Can you work these out from the model? Positions are in its coordinate system, mm. A direction names the side the tool comes from. Give positions to 0.01 mm unless a question says otherwise; leave off trailing zeros. Order: outer loops, then holes, each group sorted by start corner. A loop starts at its lowest first (then second) coordinate and runs counter-clockwise, first axis right, second up. Notation, with made-up numbers: (10.25, -27) - (22.25, -27) arc R17 cw to (22.25, -22) - close; hole circle Ø10 at (-7.75, -37.5). An arc over 180 degrees is marked (long way). Return JSON: item names as keys, results as strings.
```python
from build123d import *

# Parameters (mm, degrees)
SKETCH1_R           = 15
BOSS_EXTRUDE1_DEPTH = 6
SKETCH5_R           = 5.35
CUT_EXTRUDE2_DEPTH  = 11.5
CUT_EXTRUDE3_START  = -1
CUT_EXTRUDE3_DEPTH  = 3
SKETCH7_R           = 3.2
CUT_EXTRUDE4_DEPTH  = 2.5


with BuildPart() as part:
    # Sketch1 → Boss-Extrude1 (new body)
    with BuildSketch(Plane(origin=(0, 0, 0), x_dir=(0, 1, 0), z_dir=(0, 0, 1))):
        with Locations(Location((0, 0, 0), (0, 0, 270))):
            Circle(SKETCH1_R)
    extrude(amount=BOSS_EXTRUDE1_DEPTH)

    # Sketch5 → Cut-Extrude2 (cut)
    with BuildSketch(Plane(origin=(0, 0, 0), x_dir=(1, 0, 0), z_dir=(0, 0, -1))):
        with Locations(Location((0, 0, 0), (0, 0, 180))):
            Circle(SKETCH5_R)
    extrude(amount=-CUT_EXTRUDE2_DEPTH, mode=Mode.SUBTRACT)

    # Sketch2 → Cut-Extrude3 (cut)
    with BuildSketch(Plane.XY.offset(6).offset(CUT_EXTRUDE3_START)):
        Polygon((8.873853267, -8.742858672), (12.008464346, -6.786446977), (11.881467657, -3.093588305), (8.619859889, -1.357141328), (5.485248811, -3.313553023), (5.6122455, -7.006411695), align=None)
        Polygon((3.134611078, 12.056411695), (-0.126996689, 13.792858672), (-3.261607767, 11.836446977), (-3.134611078, 8.143588305), (0.126996689, 6.407141328), (3.261607767, 8.363553023), align=None)
        Polygon((-12.008464346, -3.313553023), (-11.881467657, -7.006411695), (-8.619859889, -8.742858672), (-5.485248811, -6.786446977), (-5.6122455, -3.093588305), (-8.873853267, -1.357141328), align=None)
    extrude(amount=-CUT_EXTRUDE3_DEPTH, mode=Mode.SUBTRACT)

    # Sketch7 → Cut-Extrude4 (cut)
    with BuildSketch(Plane.XY.offset(6)):
        with Locations((8.746856578, -5.05)):
            Circle(SKETCH7_R)
        with Locations((0, 10.1)):
            Circle(SKETCH7_R)
        with Locations((-8.746856578, -5.05)):
            Circle(SKETCH7_R)
    extrude(amount=-CUT_EXTRUDE4_DEPTH, mode=Mode.SUBTRACT)


solid = part.part
```
1. For pin 1 Ø3 at (x, z) = (-4.5, 4.5) entering from +Y; pin 2 Ø3 at (x, z) = (-8.5, 1) entering from -Y; pin 3 Ø2 at (y, z) = (-11.5, 3) entering from -X, each with a flat end and sliding along its axis, tell me the tip position at first contact or that it passes through.
Checks:
{"pin 1": "y = 14.7", "pin 2": "y = -13.27", "pin 3": "x = -10.71"}
2. Suppose I cut it at B-B (z = 5.55). List the corners of the cut face in (x, y) for me, plus the area to 3 significant figures.
Checks:
{"outline": "circle Ø30 at (0, 0); hole circle Ø6.4 at (-8.75, -5.05); hole circle Ø10.7 at (0, 0); hole circle Ø6.4 at (0, 10.1); hole circle Ø6.4 at (8.75, -5.05)", "area": "520 mm^2"}
3. Suppose I cut it at D-D (x = -6). List the corners of the cut face in (y, z) for me, plus the area to 3 significant figures.
Checks:
{"outline": "(-13.75, 0) - (13.75, 0) - (13.75, 6) - (-3.41, 6) - (-3.41, 5) - (-2.89, 5) - (-2.89, 2) - (-7.11, 2) - (-7.11, 5) - (-6.69, 5) - (-6.69, 6) - (-13.75, 6) - close", "area": "149 mm^2"}
4. Suppose I cut it at C-C (x = 1). List the corners of the cut face in (y, z) for me.
Checks:
{"outline": "(-14.97, 0) - (-5.26, 0) - (-5.26, 6) - (-14.97, 6) - close; (5.26, 0) - (14.97, 0) - (14.97, 6) - (13.14, 6) - (13.14, 5) - (13.19, 5) - (13.19, 2) - (6.95, 2) - (6.95, 5) - (7.06, 5) - (7.06, 6) - (5.26, 6) - close"}
5. Suppose I cut it at A-A (y = 0). List the corners of the cut face in (x, z) for me.
Checks:
{"outline": "(-15, 0) - (-5.35, 0) - (-5.35, 6) - (-15, 6) - close; (5.35, 0) - (15, 0) - (15, 6) - (5.35, 6) - close"}
6. If I drill on L1, parallel to Y at x = 0, z = 5.35; L2, parallel to Y at x = 0, z = 1.8; L3, parallel to Y at x = 0, z = 2.3, over which ranges is the centre line in solid material (lowest first)? Write a range as [from, to].
Checks:
{"L1": "[-15, -5.35], [5.35, 6.9], [13.3, 15]", "L2": "[-15, -5.35], [5.35, 15]", "L3": "[-15, -5.35], [5.35, 6.47], [13.73, 15]"}
7. Thinking about a two-plate mould opening in Y: for faces 3 (the face through (11.7, -6.28, 5.51)), 4 (the face through (6, 0, 6)), which applies, +Y half, -Y half, draft (parallel to the pull), parting line (faces both ways), or undercut?
Checks:
{"face 3": "undercut", "face 4": "draft"}
8. On a 3-axis mill with a long thin cutter (end or side, diameter ignored), from which of +Z, -Z, +X, -X, +Y, -Y can I reach the whole of each face in a straight line? I mean faces 1 (the face through (11.6, -3.27, 5)), 2 (the face through (-0.694, 6.976, 5.507)). Say none if no direction works.
Checks:
{"face 1": "none", "face 2": "+Z"}
